The model under review builds one solid part; all positions refer to its coordinate system, in mm. A direction names the side the tool comes from. Round coordinates to 2 decimals unless told otherwise and drop trailing zeros. Write each loop counter-clockwise with the first axis right and the second up, starting at its lowest first coordinate (ties: lowest second). Pieces come first, ordered by that corner, then holes. Notation, with made-up numbers: (16.25, -3) - (48.25, -3) arc R25 ccw to (48.25, 15) - close; hole circle Ø1 at (5.25, -36.75). An arc over 180 degrees is marked (long way). Write each question's results on one line, items separated by ' | '.
```python
from build123d import *

# Parameters (mm, degrees)
SKETCH1_R             = 5
BOSS_EXTRUDE3_DEPTH   = 8
SKETCH1_R_2           = 152.5
SKETCH1_R_3           = 109
BOSS_EXTRUDE3_2_DEPTH = 8
BOSS_EXTRUDE4_DEPTH   = 23.75
SKETCH1_9_R           = 109
SKETCH1_9_R_2         = 105
BOSS_EXTRUDE5_DEPTH   = 10
BOSS_EXTRUDE6_DEPTH   = 23.75
BOSS_EXTRUDE7_START   = -8
SKETCH2_R             = 40
SKETCH2_R_2           = 5
BOSS_EXTRUDE7_DEPTH   = 8
FILLET1_R             = 20


with BuildPart() as part:
    # Sketch1 → Boss-Extrude3 (new body)
    with BuildSketch(Plane(origin=(0, 0, 0), x_dir=(1, 0, 0), z_dir=(0, 1, 0))):
        with BuildLine():
            ThreePointArc((10, 104.522724802), (0, 105), (-10, 104.522724802))
            Line((-10, 104.522724802), (-10, 10))
            Line((-10, 10), (-104.522724802, 10))
            ThreePointArc((-104.522724802, 10), (-105, 0), (-104.522724802, -10))
            Line((-104.522724802, -10), (-10, -10))
            Line((-10, -10), (-10, -104.522724802))
            ThreePointArc((-10, -104.522724802), (0, -105), (10, -104.522724802))
            Line((10, -104.522724802), (10, -10))
            Line((10, -10), (104.522724802, -10))
            ThreePointArc((104.522724802, -10), (105, 0), (104.522724802, 10))
            Line((104.522724802, 10), (10, 10))
            Line((10, 10), (10, 104.522724802))
        make_face()
        with Locations(Location((0, 0, 0), (0, 0, 270))):
            Circle(SKETCH1_R, mode=Mode.SUBTRACT)
    extrude(amount=BOSS_EXTRUDE3_DEPTH)



with BuildPart() as body_2:
    # Sketch1 → Boss-Extrude3 2 (new body)
    with BuildSketch(Plane(origin=(0, 0, 0), x_dir=(1, 0, 0), z_dir=(0, 1, 0))):
        with Locations(Location((0, 0, 0), (0, 0, 270))):
            Circle(SKETCH1_R_2)
        with Locations(Location((0, 0, 0), (0, 0, 270))):
            Circle(SKETCH1_R_3, mode=Mode.SUBTRACT)
    extrude(amount=BOSS_EXTRUDE3_2_DEPTH)

    # Sketch1<8> → Boss-Extrude4 (add)
    with BuildSketch(Plane(origin=(0, 0, 0), x_dir=(1, 0, 0), z_dir=(0, 1, 0))):
        with BuildLine():
            Line((25, 154.490290957), (25, 150.436863833))
            ThreePointArc((25, 150.436863833), (116.337332787, 98.599568965), (152.5, 0))
            ThreePointArc((152.5, 0), (12.667954727, -151.972934837), (-150.395382597, -25.248344371))
            Line((-150.395382597, -25.248344371), (-154.44989837, -25.248344371))
            ThreePointArc((-154.44989837, -25.248344371), (110.751132294, -110.573218709), (25, 154.490290957))
        make_face()
    extrude(amount=BOSS_EXTRUDE4_DEPTH)


with BuildPart() as part_1:
    add(part.part)

    add(body_2.part)  # Boss-Extrude5 merges body 2
    # Sketch1<9> → Boss-Extrude5 (add)
    with BuildSketch(Plane(origin=(0, 0, 0), x_dir=(1, 0, 0), z_dir=(0, 1, 0))):
        with Locations(Location((0, 0, 0), (0, 0, 270))):
            Circle(SKETCH1_9_R)
        with Locations(Location((0, 0, 0), (0, 0, 84.5349762))):
            Circle(SKETCH1_9_R_2, mode=Mode.SUBTRACT)
    extrude(amount=BOSS_EXTRUDE5_DEPTH)

    # Sketch1<10> → Boss-Extrude6 (add)
    with BuildSketch(Plane(origin=(0, 0, 0), x_dir=(1, 0, 0), z_dir=(0, 1, 0))):
        with BuildLine():
            ThreePointArc((-150.395382597, 25.248344371), (-107.744727994, 107.922766781), (-25, 150.436863833))
            Line((-25, 150.436863833), (-25, 154.490290957))
            ThreePointArc((-25, 154.490290957), (-110.573218709, 110.751132294), (-154.44989837, 25.248344371))
            Line((-154.44989837, 25.248344371), (-150.395382597, 25.248344371))
        make_face()
    extrude(amount=BOSS_EXTRUDE6_DEPTH)

    # Sketch2 → Boss-Extrude7 (add)
    with BuildSketch(Plane(origin=(0, 8, 0), x_dir=(1, 0, 0), z_dir=(0, 1, 0)).offset(BOSS_EXTRUDE7_START)):
        Circle(SKETCH2_R)
        with Locations(Location((0, 0, 0), (0, 0, 270))):
            Circle(SKETCH2_R_2, mode=Mode.SUBTRACT)
    extrude(amount=BOSS_EXTRUDE7_DEPTH)

    # Fillet1
    # the kernel refuses this fillet: 20 mm, written as the material it adds along each edge
    with BuildSketch(Plane(origin=(-38.729833462, 8, 10), x_dir=(-1, 0, 0), z_dir=(0, -1, 0)), Plane(origin=(10, 8, 38.729833462), x_dir=(0, 0, 1), z_dir=(0, -1, 0)), Plane(origin=(-10, 8, -38.729833462), x_dir=(0, 0, -1), z_dir=(0, -1, 0)), Plane(origin=(38.729833462, 8, -10), x_dir=(1, 0, 0), z_dir=(0, -1, 0))) as fillet1_piece_1:
        with BuildLine():
            CenterArc((13.231690765, -20), FILLET1_R, 90, 60)
            ThreePointArc((-4.088817311, -10), (-1.705241726, -5.138679161), (0, 0))
            Line((0, 0), (13.231690765, 0))
        make_face()
    extrude(amount=8)
    with BuildSketch(Plane(origin=(-38.729833462, 8, -10), x_dir=(-1, 0, 0), z_dir=(0, -1, 0)), Plane(origin=(-10, 8, 38.729833462), x_dir=(0, 0, 1), z_dir=(0, -1, 0)), Plane(origin=(38.729833462, 8, 10), x_dir=(1, 0, 0), z_dir=(0, -1, 0)), Plane(origin=(10, 8, -38.729833462), x_dir=(0, 0, -1), z_dir=(0, -1, 0))) as fillet1_piece_2:
        with BuildLine():
            CenterArc((13.231690765, 20), FILLET1_R, 210, 60)
            ThreePointArc((-4.088817311, 10), (-1.705241726, 5.138679161), (0, 0))
            Line((0, 0), (13.231690765, 0))
        make_face()
    extrude(amount=8)
    with BuildSketch(Plane(origin=(-10, 0, -104.522724802), x_dir=(-0.974109622021504, 0, 0.22607619132744317), z_dir=(0, 1, 0)), Plane(origin=(104.522724802, 0, -10), x_dir=(-0.22607619132744408, 0, -0.9741096220215036), z_dir=(0, 1, 0)), Plane(origin=(10, 0, 104.522724802), x_dir=(0.9741096220215038, 0, -0.2260761913274436), z_dir=(0, 1, 0)), Plane(origin=(-104.522724802, 0, 10), x_dir=(0.22607619132744342, 0, 0.974109622021504), z_dir=(0, 1, 0))) as fillet1_piece_3:
        with BuildLine():
            CenterArc((25.13248218, 19.824257879), FILLET1_R, 166.933829853, 110.667316494)
            Line((5.65028974, 24.345781705), (0, 0))
            ThreePointArc((0, 0), (13.88900331, -0.922646137), (27.77800662, 0))
        make_face()
    extrude(amount=8)
    with BuildSketch(Plane(origin=(10, 0, -104.522724802), x_dir=(0.974109622021504, 0, 0.2260761913274437), z_dir=(0, 1, 0)), Plane(origin=(104.522724802, 0, 10), x_dir=(-0.22607619132744344, 0, 0.9741096220215039), z_dir=(0, 1, 0)), Plane(origin=(-10, 0, 104.522724802), x_dir=(-0.9741096220215041, 0, -0.22607619132744258), z_dir=(0, 1, 0)), Plane(origin=(-104.522724802, 0, -10), x_dir=(0.22607619132744275, 0, -0.9741096220215041), z_dir=(0, 1, 0))) as fillet1_piece_4:
        with BuildLine():
            CenterArc((25.13248218, -19.824257879), FILLET1_R, 82.398853653, 110.667316494)
            Line((5.65028974, -24.345781705), (0, 0))
            ThreePointArc((0, 0), (13.88900331, 0.922646137), (27.77800662, 0))
        make_face()
    extrude(amount=8)


solid = part_1.part
```
Q1. We need section A-A (x = 0). State the section outline as (y, z) points.
Evaluation:
outline: (0, -152.5) - (8, -152.5) - (8, -109) - (10, -109) - (10, -105) - (8, -105) - (8, -5) - (0, -5) - close; (0, 5) - (8, 5) - (8, 105) - (10, 105) - (10, 109) - (8, 109) - (8, 152.5) - (23.75, 152.5) - (23.75, 156.5) - (0, 156.5) - close
Q2. For probe 1 along X at (y, z) = (2.5, 0); probe 2 along Z at (x, y) = (-68.5, 4.5); probe 3 along X at (y, z) = (1.75, -24), list the stretches that pass through material, from the lowest coordinate up.
Evaluation:
probe 1: x = -152.5 to -5, 5 to 156.5 | probe 2: z = -140.71 to -79.58, -10 to 10, 79.58 to 140.71 | probe 3: x = -150.6 to -98.61, -32 to 32, 98.61 to 154.65
Q3. We need section C-C (z = -127). State the section outline as (x, y) points, plus the area to 3 significant figures.
Evaluation:
outline: (-91.45, 0) - (91.45, 0) - (91.45, 23.75) - (84.42, 23.75) - (84.42, 8) - (-84.42, 8) - (-84.42, 23.75) - (-91.45, 23.75) - close | area: 1,680 mm^2
Q4. Tool access review of faces 4 (the cylindrical face through (-106.408, 8.986, -23.629)), 5 (the flat face through (-5, 0, 32)), 6 (the cylindrical face through (12.6, 4.1, 42.1)): name each direction out of +Z, -Z, +X, -X, +Y, -Y from which nothing blocks a thin tool from reaching the whole face with its end or side.
Evaluation:
face 4: +Y | face 5: +Z, -Z, +X, -X, -Y | face 6: +Y, -Y
Q5. The part is to be moulded in two halves that separate along X. For faces 1 (the flat face through (115, 23.75, 104)), 2 (the cylindrical face through (-152.5, 3.9, -0.4)), 3 (the flat face through (89, 10, -57)), say which applies: released by +X, released by -X, zero draft, split by the parting line, or undercut.
Evaluation:
face 1: zero draft | face 2: released by -X | face 3: undercut
Q6. Insertion check: P1, Ø4, axis at y = 8.5, z = 23.5, coming from the +X side; P2, Ø10, axis at x = 68.5, y = 15, coming from the -Z side; P3, Ø5, axis at y = 21, z = 123, coming from the +X side; P4, Ø6, axis at x = 0, z = 0, coming from the +Y side. Each pin has a flat end and moves straight along its axis. Give the tip position at first contact, or say it passes through.
Evaluation:
P1: stops at x = 155.02 | P2: stops at z = -143.04 | P3: stops at x = 99.86 | P4: passes through
Q7. We need section B-B (x = -94). State the section outline as (y, z) points, plus the area to 3 significant figures.
Evaluation:
outline: (0, -125.12) - (23.75, -125.12) - (23.75, -120.08) - (8, -120.08) - (8, -55.18) - (10, -55.18) - (10, -46.79) - (0, -46.79) - close; (0, -16.19) - (8, -16.19) - (8, 16.19) - (0, 16.19) - close; (0, 46.79) - (10, 46.79) - (10, 55.18) - (8, 55.18) - (8, 120.08) - (23.75, 120.08) - (23.75, 125.12) - (0, 125.12) - close | area: 1,700 mm^2
Q8. We need section D-D (x = 46.5). State the section outline as (y, z) points, plus the area to 3 significant figures.
Evaluation:
outline: (0, -149.43) - (23.75, -149.43) - (23.75, -145.24) - (8, -145.24) - (8, -98.58) - (10, -98.58) - (10, -94.14) - (0, -94.14) - close; (0, -10.76) - (8, -10.76) - (8, 10.76) - (0, 10.76) - close; (0, 94.14) - (10, 94.14) - (10, 98.58) - (8, 98.58) - (8, 145.24) - (23.75, 145.24) - (23.75, 149.43) - (0, 149.43) - close | area: 1,210 mm^2
